Check sheet for the drawn part. Datum: minimum x, y, z corner. Units: mm. A direction names the side the tool comes from. Give positions to 0.01 mm unless a question says otherwise; leave off trailing zeros. Order: outer loops, then holes, each group sorted by start corner. A loop starts at its lowest first (then second) coordinate and runs counter-clockwise, first axis right, second up.
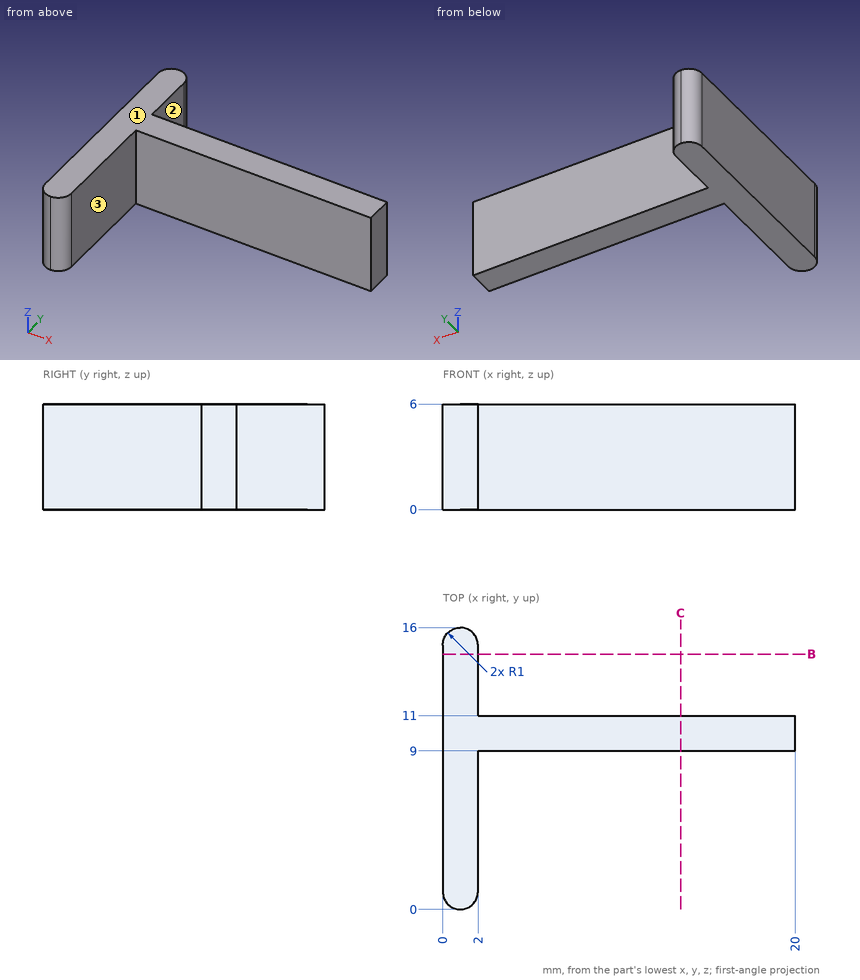
(1) Scan lines: line 1 (X direction, y = 5.5, z = 5.25); line 2 (Y direction, x = 10.75, z = 0.4). Record each from-to range of solid material in increasing order.
Solved:
line 1: x = 0 to 2
line 2: y = 9 to 11
(2) Set-up check for the marked faces 1, 2 and 3: record each of +Z, -Z, +X, -X, +Y, -Y from which the full face is reachable in a straight line by a thin tool's end or side.
Solved:
face 1: +Z, +X, -X, +Y, -Y
face 2: +Z, -Z, +X, +Y
face 3: +Z, -Z, +X, -Y
(3) Go/stop test with flat-tipped pins: pin 1 (1.2 mm diameter, centred on y = 12.5, z = 3.5, fed in from +X); pin 2 (1.5 mm diameter, centred on x = 4, z = 5.5, fed in from -Y). Record where each tip stops, or that it passes through.
Solved:
pin 1: stops at x = 2
pin 2: stops at y = 9
(4) Section check B-B, the plane y = 14.5. Enter the section's corners in (x, z).
Solved:
outline: (0, 0) - (2, 0) - (2, 6) - (0, 6) - close
(5) Section check C-C, the plane x = 13.5. Enter the section's corners in (y, z).
Solved:
outline: (9, 0) - (11, 0) - (11, 6) - (9, 6) - close
